Verification items for the finished model (mm, model axes). A direction names the side the tool comes from. Round coordinates to 2 decimals unless told otherwise and drop trailing zeros. Write each loop counter-clockwise with the first axis right and the second up, starting at its lowest first coordinate (ties: lowest second). Pieces come first, ordered by that corner, then holes. Notation, with made-up numbers: M 3,-27.5 L 7,-27.5 A19 cw 7,-20.5 Z; hole C 81.25,83 d1. An arc over 180 degrees is marked long. Answer in a Markdown table with one row per item. Add a question column.
1. Set-up check for faces 4 (the flat face through (-3, 0, 2)), 5 (the flat face through (9.5, -9.5, 0)), 6 (the cylindrical face through (2.579, 1.978, 7.331)): record each of +Z, -Z, +X, -X, +Y, -Y from which the full face is reachable in a straight line by a thin tool's end or side.
2. Go/stop test with flat-tipped pins: pin 1 Ø2 at (x, z) = (17, 1.5) entering from +Y; pin 2 Ø2 at (y, z) = (-13, 6.5) entering from +X; pin 3 Ø1.5 at (x, y) = (11, 7) entering from -Z; pin 4 Ø1.8 at (x, y) = (14.45, 0) entering from +Z. Record where each tip stops, or that it passes through.
3. Sectioned sample at B-B on y = 0. Record the cut outline in (x, z).
4. Material ranges on probe 1 along Y at (x, z) = (0, 1.75); probe 2 along Y at (x, z) = (-14.45, 1.35); probe 3 along Z at (x, y) = (11.5, 16), recorded low to high.
5. Draft check along Y on faces 1 (the cylindrical face through (-4.769, -21.477, 2.958)), 2 (the conical face through (-0.36, -18.61, 3.15)), 3 (the flat face through (5, 0, 6)). Enter one of: pulls with the +Y half, pulls with the -Y half, needs draft (parallel to the pull), parting line crosses it, or undercut.
6. Sectioned sample at C-C on z = 5. Record the cut outline in (x, y), plus the area to 3 significant figures.
7. Sectioned sample at A-A on x = 0. Record the cut outline in (y, z).
8. Sectioned sample at D-D on y = -17. Record the cut outline in (x, z).
```python
from build123d import *

# Parameters (mm, degrees)
SKETCH_1_R          = 22
EXTRUDE_1_DEPTH     = 6
SKETCH_2_R          = 3.25
EXTRUDE_2_DEPTH     = 2.7
SKETCH_3_R          = 2.5
CUT_EXTRUDE_1_DEPTH = 33.306191357
SKETCH_4_R          = 0.8
CUT_EXTRUDE_2_DEPTH = 32.685959036
SKETCH_5_R          = 13
CUT_EXTRUDE_3_DEPTH = 2
SKETCH_6_R          = 1.5
CUT_EXTRUDE_4_DEPTH = 32.685959036
CHAMFER_1_SIZE      = 3


with BuildPart() as part:
    # Эскиз1 → Бобышка-Вытянуть1 (new body)
    with BuildSketch(Plane.XY):
        Circle(SKETCH_1_R)
    extrude(amount=EXTRUDE_1_DEPTH)

    # Эскиз2 → Бобышка-Вытянуть2 (add)
    with BuildSketch(Plane.XY.offset(6)):
        with Locations(Location((0, 0, 0), (0, 0, 180))):
            Circle(SKETCH_2_R)
    extrude(amount=EXTRUDE_2_DEPTH)

    # Эскиз3 → Вырез-Вытянуть1 (cut, through all)
    with BuildSketch(Plane.XY.offset(8.7)):
        Circle(SKETCH_3_R)
    extrude(amount=-CUT_EXTRUDE_1_DEPTH, mode=Mode.SUBTRACT)

    # Эскиз4 → Вырез-Вытянуть2 (cut, through all)
    with BuildSketch(Plane.XY.offset(6)):
        with Locations((-14.45, 0)):
            Circle(SKETCH_4_R)
        with Locations((14.45, 0)):
            Circle(SKETCH_4_R)
    extrude(amount=-CUT_EXTRUDE_2_DEPTH, mode=Mode.SUBTRACT)

    # Эскиз5 → Вырез-Вытянуть3 (cut)
    with BuildSketch(Plane(origin=(0, 0, 0), x_dir=(-1, 0, 0), z_dir=(0, 0, -1))):
        Circle(SKETCH_5_R)
    extrude(amount=-CUT_EXTRUDE_3_DEPTH, mode=Mode.SUBTRACT)

    # Эскиз6 → Вырез-Вытянуть4 (cut, through all)
    with BuildSketch(Plane.XY.offset(6)):
        with Locations((0, -17)):
            Circle(SKETCH_6_R)
        with Locations((-14.722431864, 8.5)):
            Circle(SKETCH_6_R)
        with Locations((14.722431864, 8.5)):
            Circle(SKETCH_6_R)
    extrude(amount=-CUT_EXTRUDE_4_DEPTH, mode=Mode.SUBTRACT)

    # Фаска1
    chamfer_1_edges = [part.edges().sort_by_distance(p)[0] for p in [
        (-1.5, -17, 6),
        (-16.222431864, 8.5, 6),
        (13.222431864, 8.5, 6),
    ]]
    chamfer(chamfer_1_edges, length=CHAMFER_1_SIZE)


solid = part.part
```
Geometry check:
| question | item | result |
|---|---|---|
| 1 | face 4 | -Z |
| 1 | face 5 | -Z, +X, -X, +Y, -Y |
| 1 | face 6 | +Z |
| 2 | pin 1 | stops at y = 15.1 |
| 2 | pin 2 | stops at x = 18.35 |
| 2 | pin 3 | stops at z = 0 |
| 2 | pin 4 | stops at z = 6 |
| 3 | outline | M -22,0 L -15.25,0 L -15.25,6 L -22,6 Z; M -13.65,0 L -13,0 L -13,2 L -2.5,2 L -2.5,8.7 L -3.25,8.7 L -3.25,6 L -13.65,6 Z; M 2.5,2 L 13,2 L 13,0 L 13.65,0 L 13.65,6 L 3.25,6 L 3.25,8.7 L 2.5,8.7 Z; M 15.25,0 L 22,0 L 22,6 L 15.25,6 Z |
| 4 | probe 1 | y = -22 to -18.5, -15.5 to -13, 13 to 22 |
| 4 | probe 2 | y = -16.59 to -0.8, 0.8 to 7.02, 9.98 to 16.59 |
| 4 | probe 3 | z = 0 to 6 |
| 5 | face 1 | parting line crosses it |
| 5 | face 2 | undercut |
| 5 | face 3 | needs draft |
| 6 | outline | C 0,0 d44; hole C -14.72,8.5 d7; hole C -14.45,0 d1.6; hole C 0,-17 d7; hole C 0,0 d5; hole C 14.72,8.5 d7; hole C 14.45,0 d1.6 |
| 6 | area | 1,380 mm2 |
| 7 | outline | M -22,0 L -18.5,0 L -18.5,3 L -21.5,6 L -22,6 Z; M -15.5,0 L -13,0 L -13,2 L -2.5,2 L -2.5,8.7 L -3.25,8.7 L -3.25,6 L -12.5,6 L -15.5,3 Z; M 2.5,2 L 13,2 L 13,0 L 22,0 L 22,6 L 3.25,6 L 3.25,8.7 L 2.5,8.7 Z |
| 8 | outline | M -13.96,0 L -1.5,0 L -1.5,3 L -4.5,6 L -13.96,6 Z; M 1.5,0 L 13.96,0 L 13.96,6 L 4.5,6 L 1.5,3 Z |
